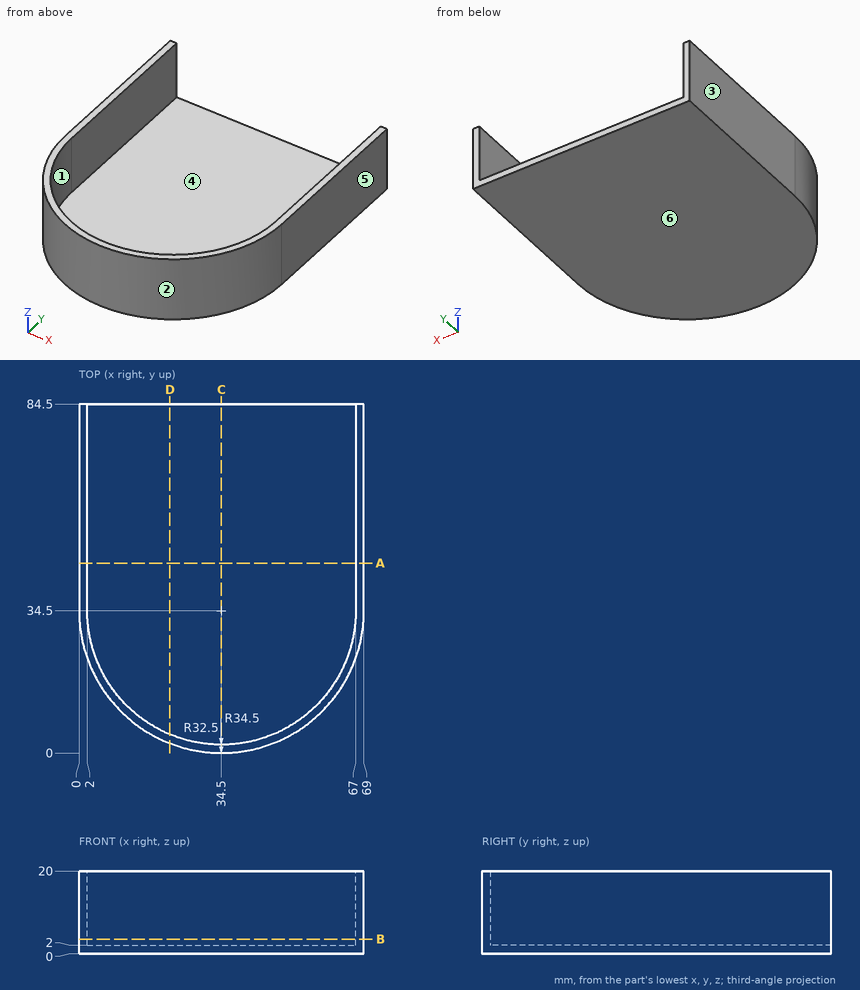
Input: dimensioned drawing with shaded views. Units: mm. Origin: part minimum x, y, z. A direction names the side the tool comes from. Round coordinates to 2 decimals unless told otherwise and drop trailing zeros. Order: outer loops, then holes, each group sorted by start corner. A loop starts at its lowest first (then second) coordinate and runs counter-clockwise, first axis right, second up.
Q1. Mould query, pull axis X, two halves, no side actions, for the marked faces 3, 4, 5 and 6. Classes: released by +X, released by -X, zero draft, split by the parting line, or undercut.
Result sheet:
face 3: released by -X
face 4: undercut
face 5: released by +X
face 6: zero draft
Q2. Pin query (flat end, axial travel): pin 1 (10 mm diameter, centred on y = 30, z = 3, fed in from +X); pin 2 (12 mm diameter, centred on x = 57, z = 10, fed in from +Y); pin 3 (8 mm diameter, centred on x = 8.5, y = 24, fed in from +Z); pin 4 (8 mm diameter, centred on x = 42, z = 4.5, fed in from -Y). Return the tip coordinate at first contact, or that it passes through.
Result sheet:
pin 1: stops at x = 69
pin 2: stops at y = 18.88
pin 3: stops at z = 2
pin 4: stops at y = 0.18
Q3. Section C-C, the plane x = 34.5. Output: boundary loops of the cut face in (y, z), and give its area (3 significant figures).
Result sheet:
outline: (0, 0) - (84.5, 0) - (84.5, 2) - (2, 2) - (2, 20) - (0, 20) - close
area: 205 mm2
Q4. Material intervals for probe 1 along X at (y, z) = (65.5, 9); probe 2 along Z at (x, y) = (63, 71.5); probe 3 along X at (y, z) = (14, 4), sorted ascending.
Result sheet:
probe 1: x = 0 to 2, 67 to 69
probe 2: z = 0 to 2
probe 3: x = 6.75 to 9.28, 59.72 to 62.25
Q5. Section B-B, the plane z = 3.5. Output: boundary loops of the cut face in (x, y).
Result sheet:
outline: (0, 34.5) arc R34.5 ccw to (69, 34.5) - (69, 84.5) - (67, 84.5) - (67, 34.5) arc R32.5 cw to (2, 34.5) - (2, 84.5) - (0, 84.5) - close
Q6. Section A-A, the plane y = 46. Output: boundary loops of the cut face in (x, z).
Result sheet:
outline: (0, 0) - (69, 0) - (69, 20) - (67, 20) - (67, 2) - (2, 2) - (2, 20) - (0, 20) - close
Q7. Section D-D, the plane x = 22. Output: boundary loops of the cut face in (y, z), and give its area (3 significant figures).
Result sheet:
outline: (2.34, 0) - (84.5, 0) - (84.5, 2) - (4.5, 2) - (4.5, 20) - (2.34, 20) - close
area: 203 mm2
Q8. Access query for the marked faces 1 and 2. Directions: +Z, -Z, +X, -X, +Y, -Y. A direction counts if a zero-diameter tool reaches every point of the face in a straight line with its end or side. Return the directions, or none.
Result sheet:
face 1: +Z, +Y
face 2: +Z, -Z, -Y
